Build history of the part. All positions in model axes, mm. Face numbers are marked on the shaded views. A direction names the side the tool comes from. Round coordinates to 2 decimals unless told otherwise and drop trailing zeros. Write each loop counter-clockwise with the first axis right and the second up, starting at its lowest first coordinate (ties: lowest second). Pieces come first, ordered by that corner, then holes. Notation, with made-up numbers: M 75,61 L 82,61 A16 cw 82,72 Z; hole C 38,-23.5 d9. An arc over 180 degrees is marked long. Write item = value, one per line.
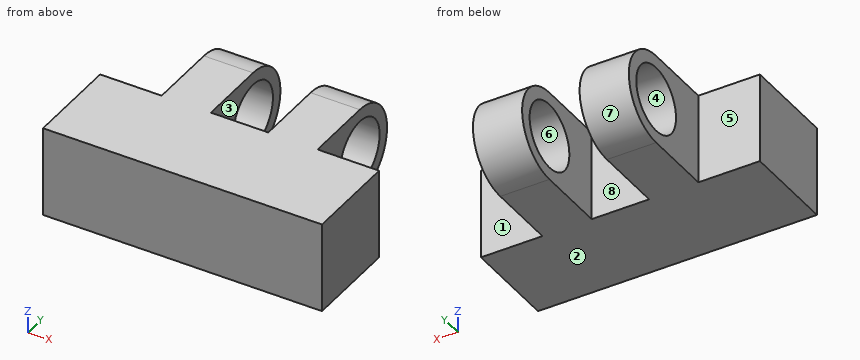
from build123d import *

# Parameters (mm, degrees)
SKETCH_1_R          = 4
EXTRUDE_1_DEPTH     = 34
SKETCH_2_W          = 7.5
SKETCH_2_H          = 14
SKETCH_2_W_2        = 3.5
CUT_EXTRUDE_2_DEPTH = 41.951190459


with BuildPart() as part:
    # 草图1 → 凸台-拉伸1 (new body)
    with BuildSketch(Plane(origin=(0, 0, 0), x_dir=(0, 0, -1), z_dir=(1, 0, 0))):
        with BuildLine():
            Line((-5.5, 0), (-5.5, -20))
            Line((-5.5, -20), (5.5, -20))
            Line((5.5, -20), (5.5, 0))
            ThreePointArc((5.5, 0), (0, 5.5), (-5.5, 0))
        make_face()
        Circle(SKETCH_1_R, mode=Mode.SUBTRACT)
    extrude(amount=EXTRUDE_1_DEPTH)

    # 草图2 → 切除-拉伸2 (cut, through all)
    with BuildSketch(Plane.XY.offset(5.5)):
        with Locations((3.75, -1.5)):
            Rectangle(SKETCH_2_W, SKETCH_2_H)
        with Locations((18.75, -1.5)):
            Rectangle(SKETCH_2_W_2, SKETCH_2_H)
        with Locations((15.25, -1.5)):
            Rectangle(SKETCH_2_W_2, SKETCH_2_H)
        with Locations((30.25, -1.5)):
            Rectangle(SKETCH_2_W, SKETCH_2_H)
    extrude(amount=-CUT_EXTRUDE_2_DEPTH, mode=Mode.SUBTRACT)


solid = part.part
1. Flat gauge pins, fed straight in: pin 1 (2 mm diameter, centred on x = 15.5, z = 2, fed in from +Y); pin 2 (5.5 mm diameter, centred on y = -4.5, z = -0.5, fed in from -X); pin 3 (5.5 mm diameter, centred on y = 1.5, z = -0.5, fed in from +X); pin 4 (5 mm diameter, centred on x = 16.5, y = -3.5, fed in from +Z). Where does each tip first touch, or does it go through?
Responses:
pin_1 = -8.5
pin_2 = 7.5
pin_3 = 26.5
pin_4 = through
2. Mould opens along Z. For the marked faces 6, 7 and 8 say: pulls with the +Z half, pulls with the -Z half, needs draft (parallel to the pull), parting line crosses it, or undercut.
Responses:
face_6 = undercut
face_7 = parting line crosses it
face_8 = needs draft
3. Probe probe 1 along X at (y, z) = (-7.5, 0); probe 2 along Y at (x, z) = (11.35, 0); probe 3 along Z at (x, y) = (10.45, 0). List the from-to ranges inside material, lowest first.
Responses:
probe_1 = 7.5 to 13.5, 20.5 to 26.5
probe_2 = -20 to -4, 4 to 5.5
probe_3 = -5.5 to -4, 4 to 5.5
4. Band-saw the part on C-C (y = -3.5). List the corners of the cut face in (x, z), plus the area to 3 significant figures.
Responses:
outline = M 7.5,-5.5 L 13.5,-5.5 L 13.5,-1.94 L 7.5,-1.94 Z; M 7.5,1.94 L 13.5,1.94 L 13.5,5.5 L 7.5,5.5 Z; M 20.5,-5.5 L 26.5,-5.5 L 26.5,-1.94 L 20.5,-1.94 Z; M 20.5,1.94 L 26.5,1.94 L 26.5,5.5 L 20.5,5.5 Z
area = 85.5 mm²
5. Band-saw the part on B-B (x = 21). List the corners of the cut face in (y, z), plus the area to 3 significant figures.
Responses:
outline = M -20,-5.5 L 0,-5.5 A5.5 ccw 0,5.5 L -20,5.5 Z; hole C 0,0 d8
area = 217 mm²
6. Band-saw the part on D-D (z = 4.5). List the corners of the cut face in (x, y).
Responses:
outline = M 0,-20 L 34,-20 L 34,-8.5 L 26.5,-8.5 L 26.5,3.16 L 20.5,3.16 L 20.5,-8.5 L 13.5,-8.5 L 13.5,3.16 L 7.5,3.16 L 7.5,-8.5 L 0,-8.5 Z
7. Tool access for the marked faces 1, 2, 3, 4 and 5: list every direction of +Z, -Z, +X, -X, +Y, -Y with a clear straight run to the whole face (end or side of a thin tool).
Responses:
face_1 = +Z, -Z, +X, +Y
face_2 = -Z, +X, -X, +Y, -Y
face_3 = +Z, -Z, +Y
face_4 = +X, -X
face_5 = +Z, -Z, -X, +Y
8. Band-saw the part on A-A (z = 0). List the corners of the cut face in (x, y), plus the area to 3 significant figures.
Responses:
outline = M 0,-20 L 34,-20 L 34,-8.5 L 26.5,-8.5 L 26.5,-4 L 20.5,-4 L 20.5,-8.5 L 13.5,-8.5 L 13.5,-4 L 7.5,-4 L 7.5,-8.5 L 0,-8.5 Z; M 7.5,4 L 13.5,4 L 13.5,5.5 L 7.5,5.5 Z; M 20.5,4 L 26.5,4 L 26.5,5.5 L 20.5,5.5 Z
area = 463 mm²
